from build123d import *

# Parameters (mm, degrees)
CUT_EXTRUDE_START   = -9
SKETCH_2_R          = 3
CUT_EXTRUDE_2_DEPTH = 9


with BuildPart() as part:
    # ｽｹｯﾁ1 → 回転1 (revolve)
    with BuildSketch(Plane.XY, mode=Mode.PRIVATE) as revolve_1_sk:
        Polygon((0, 0), (0, 29), (3, 29), (3, 20), (12, 20), (12, 17), (3, 17), (3, 0), align=None)
    revolve(revolve_1_sk.sketch.rotate(Axis((0, 0, 0), (0, 1, 0)), 90), axis=Axis((0, 0, 0), (0, 1, 0)))

    # ｽｹｯﾁ2 → ｶｯﾄ - 押し出し2 (cut)
    with BuildSketch(Plane(origin=(0, 29, 0), x_dir=(1, 0, 0), z_dir=(0, 1, 0)).offset(CUT_EXTRUDE_START)):
        with Locations(Location((0, 0, 0), (0, 0, 90))):
            Circle(SKETCH_2_R)
        Polygon((1.437961457, -2.503118092), (2.886744585, -0.006247894), (1.448783128, 2.496870197), (-1.437961457, 2.503118092), (-2.886744585, 0.006247894), (-1.448783128, -2.496870197), align=None, mode=Mode.SUBTRACT)
    extrude(amount=CUT_EXTRUDE_2_DEPTH, mode=Mode.SUBTRACT)


solid = part.part
Model file for the job. Use its own axes, mm. A direction names the side the tool comes from. Round coordinates to 2 decimals unless told otherwise and drop trailing zeros. Order: outer loops, then holes, each group sorted by start corner. A loop starts at its lowest first (then second) coordinate and runs counter-clockwise, first axis right, second up. Notation, with made-up numbers: M 59.25,8 L 86.25,8 A27 cw 86.25,38 Z; hole C 4.25,-32.75 d9. An arc over 180 degrees is marked long. Write each question's results on one line, items separated by ' | '. Start each with the question number.
(1) Saw through at D-D, the plane y = 9.75. Give the cut face in (x, z), then the cut area to 3 significant figures.
(2) Which spindle directions (+Z, -Z, +X, -X, +Y, -Y) get a long thin tool onto all of the face, cutting with end or side? Do faces 1 (the face through (2.5, 17, -2.5)), 2 (the face through (2.152, 24.437, 1.272)), 3 (the face through (2.178, 24.437, -1.228)). Say none if no direction does.
(3) Probe probe 1 along Z at (x, y) = (-1.25, 22.75); probe 2 along Y at (x, z) = (9, -4.5); probe 3 along X at (y, z) = (19.5, -9). List the from-to ranges inside material, lowest first. Write a range as from..to.
(4) Drop flat-ended pins along their axis: pin 1 (1.5 mm diameter, centred on x = 5, y = 20.5, fed in from -Z); pin 2 (3 mm diameter, centred on x = 6, z = 7.5, fed in from +Y); pin 3 (3 mm diameter, centred on y = 20, z = -8.5, fed in from -X). Give the stop position or say it passes through.
(5) Saw through at A-A, the plane x = 0. Give the cut face in (y, z), then the cut area to 3 significant figures.
(6) Saw through at C-C, the plane z = -1.75. Give the cut face in (x, y), then the cut area to 3 significant figures.
(7) Saw through at B-B, the plane y = 24. Give the cut face in (x, z), then the cut area to 3 significant figures.
Established:
1) outline: C 0,0 d6 | area: 28.3 mm^2
2) face 1: -Y | face 2: +Z, +X, +Y | face 3: -Z, +X, +Y
3) probe 1: z = -2.5..2.5 | probe 2: y = 17..20 | probe 3: x = -7.94..7.94
4) pin 1: stops at z = -11.15 | pin 2: stops at y = 20 | pin 3: stops at x = -9.75
5) outline: M 0,-3 L 17,-3 L 17,-12 L 20,-12 L 20,-2.5 L 29,-2.5 L 29,2.5 L 20,2.5 L 20,12 L 17,12 L 17,3 L 0,3 Z | area: 219 mm^2
6) outline: M -11.87,17 L -2.44,17 L -2.44,0 L 2.44,0 L 2.44,17 L 11.87,17 L 11.87,20 L 1.88,20 L 1.88,29 L -1.87,29 L -1.87,20 L -11.87,20 Z | area: 188 mm^2
7) outline: M -2.89,-0.01 L -1.44,-2.5 L 1.45,-2.5 L 2.89,0.01 L 1.44,2.5 L -1.45,2.5 Z | area: 21.7 mm^2
